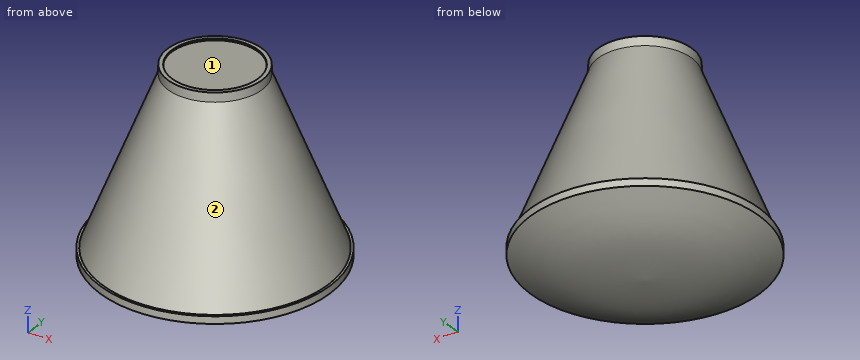
from build123d import *


# Not quite as in the source:
# - a feature of the source that left no trace in its solid (it failed there, or was rolled back) is left out


with BuildPart() as f1:
    # F0 (on Front) → F1 (revolve)
    with BuildSketch(Plane.XZ):
        with BuildLine():
            Line((11.3937472925, 47.8038191795), (0, 47.8038191795))
            Line((0, 47.8038191795), (0, -6.5516876057))
            add(Edge.make_bspline(
                [(0, -6.5516876057), (6.0146157822, -6.2971422391), (17.4152007991, -5.8146565414), (26.2624737662, -1.8656336954), (30.4421838373, 0)],
                knots=[0, 0, 0, 0, 0.5275708021, 1, 1, 1, 1], degree=3))
            Line((30.4421838373, 0), (30.4421838373, 1.9357798155))
            Line((30.4421838373, 1.9357798155), (29.8244003206, 1.9357798155))
            Line((29.8244003206, 1.9357798155), (12.4743720517, 45.8226278424))
            Line((12.4743720517, 45.8226278424), (12.4743720517, 48.2841059566))
            Line((12.4743720517, 48.2841059566), (11.3937472925, 48.2841059566))
            Line((11.3937472925, 48.2841059566), (11.3937472925, 47.8038191795))
        make_face()
    revolve(axis=Axis((0, 0, 20.6260657869), (0, 0, -1)))


solid = f1.part
Build history of the part. All positions in model axes, mm. Face numbers are marked on the shaded views. Give positions to 0.01 mm unless a question says otherwise; leave off trailing zeros. Order: outer loops, then holes, each group sorted by start corner. A loop starts at its lowest first (then second) coordinate and runs counter-clockwise, first axis right, second up. Notation, with made-up numbers: M 70.5,48.5 L 76.5,48.5 A25 ccw 76.5,72.5 Z; hole C 7.25,57 d9. An arc over 180 degrees is marked long. Put each result on its own line as item: value.
Item 1: Pull direction Y, two halves, no side cores. Call the marked faces 1 and 2: +Y half, -Y half, draft (parallel to the pull), parting line (faces both ways), or undercut.
Results are:
face 1: undercut
face 2: parting line
Item 2: Drop flat-ended pins along their axis: pin 1 Ø4 at (y, z) = (10.5, 34.5) entering from -X; pin 2 Ø4 at (x, z) = (-7.5, 41) entering from -Y; pin 3 Ø5 at (x, z) = (-15, 13.5) entering from +Y. Give the stop position or say it passes through.
Results are:
pin 1: x = -14.98
pin 2: y = -13.64
pin 3: y = 22.34
Item 3: Wall check: probe 1 along X at (y, z) = (0, 48.2); probe 2 along X at (y, z) = (0, 47). Give the ranges that are in metal, low to high.
Results are:
probe 1: -12.47 to -11.39, 11.39 to 12.47
probe 2: -12.47 to 12.47
Item 4: Cut at B-B on z = 26. Write the cut outline in (x, y).
Results are:
outline: C 0,0 d40.62
Item 5: Cut at A-A on z = 12. Write the cut outline in (x, y).
Results are:
outline: C 0,0 d51.69
